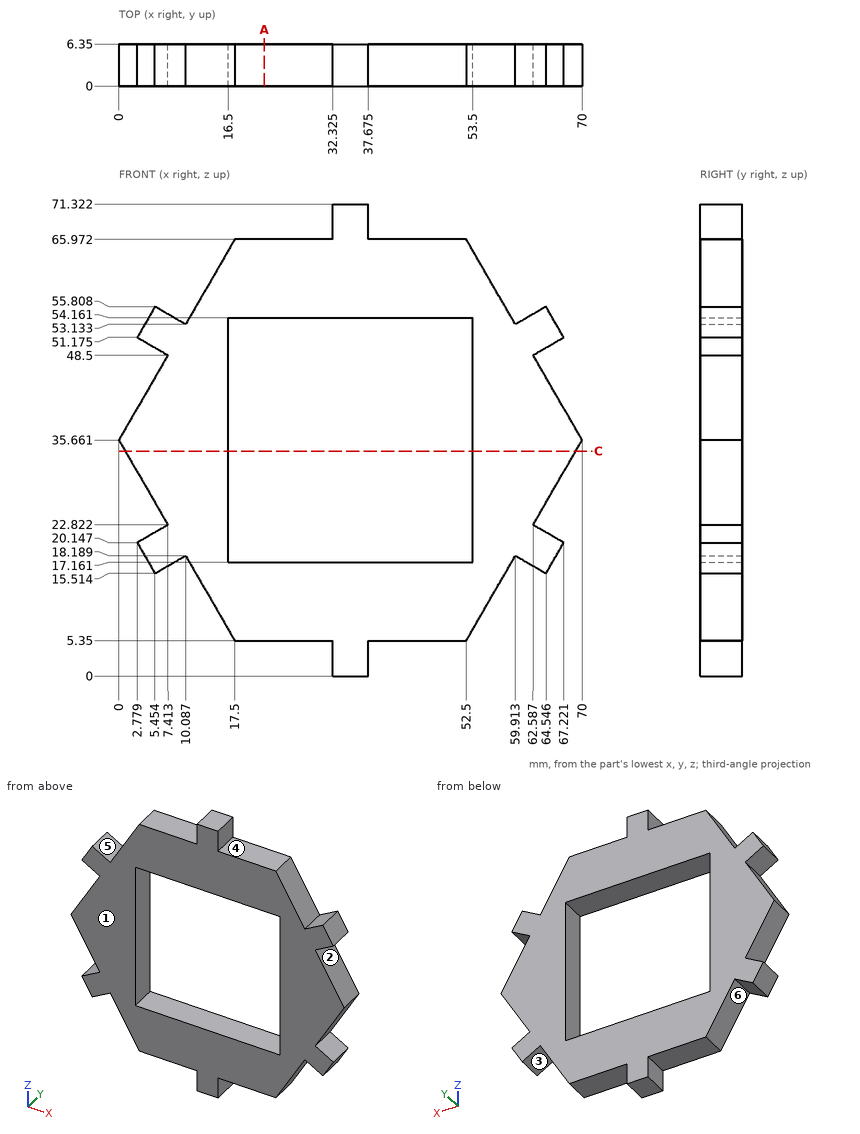
The figure shows three views and two pictorial views of one solid part (mm, origin at its lowest corner). Answer the questions. A direction names the side the tool comes from. Give positions to 0.01 mm unless a question says otherwise; leave off trailing zeros. Order: outer loops, then holes, each group sorted by start corner. A loop starts at its lowest first (then second) coordinate and runs counter-clockwise, first axis right, second up. Notation, with made-up numbers: (47.25, 39.25) -> (105.25, 39.25) arc R13 ccw to (105.25, 58.25) -> close; hole circle Ø11 at (47.5, 11.25). An arc over 180 degrees is marked (long way). Write each question's results on one line, items separated by ' | '.
Q1. Which of the six approach directions +Z, -Z, +X, -X, +Y, -Y give full straight-line access (tool end or side, diameter ignored) to the marked faces 4, 5 and 6?
Checked values:
face 4: +Z, +X, +Y, -Y | face 5: +Z, +Y, -Y | face 6: -Z, +Y, -Y
Q2. The part is cut by section A-A, the plane x = 22. Give the vertices of the cut face in (y, z).
Checked values:
outline: (0, 5.35) -> (6.35, 5.35) -> (6.35, 17.16) -> (0, 17.16) -> close; (0, 54.16) -> (6.35, 54.16) -> (6.35, 65.97) -> (0, 65.97) -> close
Q3. The part is cut by section C-C, the plane z = 34. Give the vertices of the cut face in (x, y), and give its area (3 significant figures).
Checked values:
outline: (0.96, 0) -> (16.5, 0) -> (16.5, 6.35) -> (0.96, 6.35) -> close; (53.5, 0) -> (69.04, 0) -> (69.04, 6.35) -> (53.5, 6.35) -> close | area: 197 mm^2
Q4. Determine the mould class of the marked faces 1, 2 and 3 for opening direction X: pulls with the +X half, pulls with the -X half, needs draft (parallel to the pull), parting line crosses it, or undercut.
Checked values:
face 1: needs draft | face 2: pulls with the +X half | face 3: undercut
Q5. Each of these flat-tipped pins is pushed along its axis until it touches: P1, Ø1.5, axis at y = 2, z = 37.5, coming from the -X side; P2, Ø1.9, axis at x = 26.5, y = 4.5, coming from the -Z side; P3, Ø1.9, axis at x = 43, y = 4.5, coming from the +Z side. Where does it stop, or does it pass through?
Checked values:
P1: stops at x = 0.63 | P2: stops at z = 5.35 | P3: stops at z = 65.97
Q6. Straight lines are drawn through the part: probe 1 along Z at (x, y) = (44.5, 0.5); probe 2 along Z at (x, y) = (36, 6); probe 3 along X at (y, z) = (0.75, 68.5) (1 decimal). For each, find the intervals that lie inside material, in ascending order. Write a range as from..to.
Checked values:
probe 1: z = 5.35..17.16, 54.16..65.97 | probe 2: z = 0..17.16, 54.16..71.32 | probe 3: x = 32.3..37.7
